Answer from the drawing. Dimensions are ordinates in mm from the lowest x, y and z of the part. A direction names the side the tool comes from. Coordinates: 2 decimals unless noted, no trailing zeros. Order: outer loops, then holes, each group sorted by start corner. A loop starts at its lowest first (then second) coordinate and runs counter-clockwise, first axis right, second up. Notation, with made-up numbers: (32, -3) - (71, -3) arc R24 ccw to (71, 14) - close; hole circle Ø10 at (58.5, -34). An arc over 180 degrees is marked (long way). Use a Markdown table: item, result. Add a question column.
Item 1: The part is cut by section B-B, the plane y = 175. Give the vertices of the cut face in (x, z), then the cut area to 3 significant figures.
Item 2: The part is cut by section C-C, the plane x = 65. Give the vertices of the cut face in (y, z).
Item 3: Find the intervals of material crossed by line 1 along Y through (x, z) = (190, 2); line 2 along X through (y, z) = (175, 3.75); line 3 along X through (y, z) = (315, 259), in increasing order.
Item 4: Flat-ended cylindrical pins translate along their axes: P1, Ø12, axis at x = 289, y = 289.5, coming from the +Z side; P2, Ø6, axis at y = 119.5, z = 246, coming from the +X side. Find the tip coordinate at first contact, or state that the pin passes through.
Item 5: The part is cut by section D-D, the plane z = 293.5. Give the vertices of the cut face in (x, y).
Item 6: The part is cut by section A-A, the plane x = 190. Give the vertices of the cut face in (y, z), then the cut area to 3 significant figures.
Item 7: For the marked faces 1 and 2, determine the directions among +Z, -Z, +X, -X, +Y, -Y from which every point of the face is accessible in a straight line to the end or side of a thin tool.
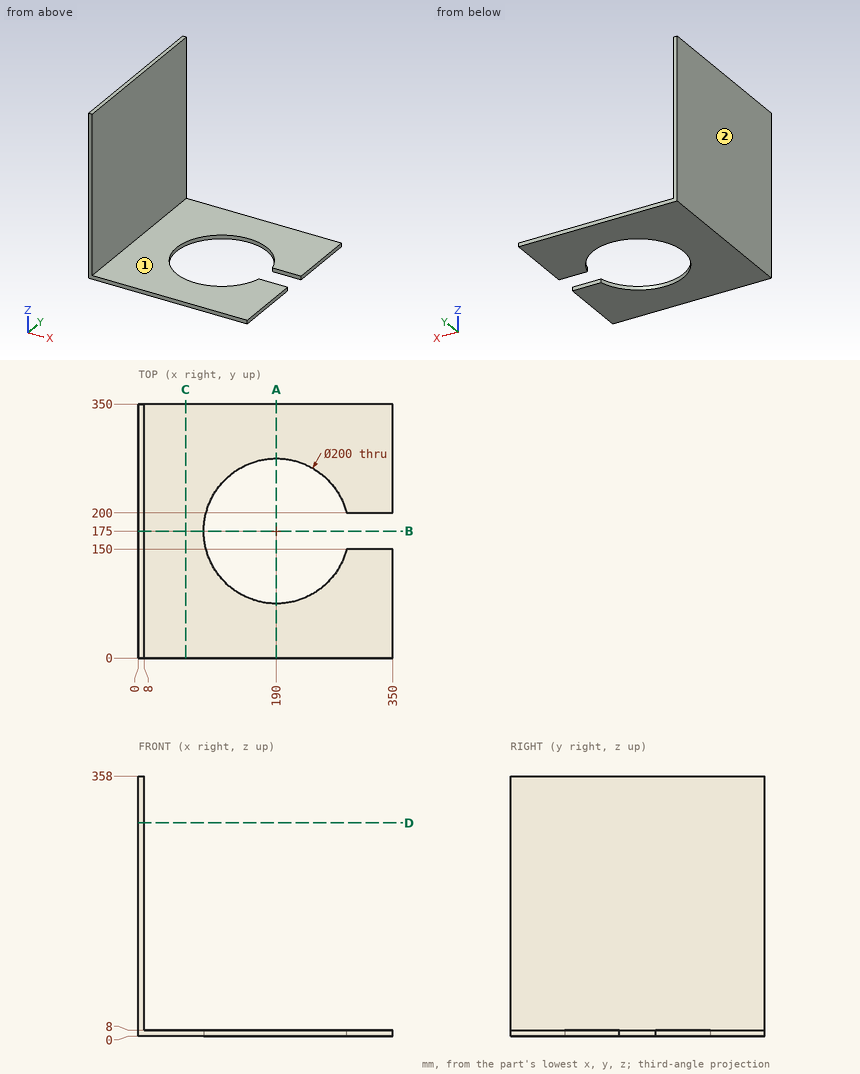
Solution:
| question | item | result |
|---|---|---|
| 1 | outline | (0, 0) - (90, 0) - (90, 8) - (8, 8) - (8, 358) - (0, 358) - close |
| 1 | area | 3,520 mm2 |
| 2 | outline | (0, 0) - (350, 0) - (350, 8) - (0, 8) - close |
| 3 | line 1 | y = 0 to 75, 275 to 350 |
| 3 | line 2 | x = 0 to 90 |
| 3 | line 3 | x = 0 to 8 |
| 4 | P1 | stops at z = 8 |
| 4 | P2 | stops at x = 8 |
| 5 | outline | (0, 0) - (8, 0) - (8, 350) - (0, 350) - close |
| 6 | outline | (0, 0) - (75, 0) - (75, 8) - (0, 8) - close; (275, 0) - (350, 0) - (350, 8) - (275, 8) - close |
| 6 | area | 1,200 mm2 |
| 7 | face 1 | +Z, +X, +Y, -Y |
| 7 | face 2 | +Z, -Z, -X, +Y, -Y |
